from build123d import *

# Parameters (mm, degrees)
SKETCH1_W           = 70.8
SKETCH1_H           = 40
BOSS_EXTRUDE1_DEPTH = 10
SKETCH2_R           = 1.32
CUT_EXTRUDE1_DEPTH  = 11
SKETCH3_R           = 3.4
CUT_EXTRUDE2_DEPTH  = 11
SKETCH4_R           = 5.375
CUT_EXTRUDE3_DEPTH  = 7


with BuildPart() as part:
    # Sketch1 → Boss-Extrude1 (new body)
    with BuildSketch(Plane.XY):
        Rectangle(SKETCH1_W, SKETCH1_H)
    extrude(amount=BOSS_EXTRUDE1_DEPTH)

    # Sketch2 → Cut-Extrude1 (cut, through all)
    with BuildSketch(Plane.XY.offset(10)):
        with Locations((15.875, -15.875)):
            Circle(SKETCH2_R)
        with Locations((-15.875, -15.875)):
            Circle(SKETCH2_R)
        with Locations((-15.875, 15.875)):
            Circle(SKETCH2_R)
        with Locations((15.875, 15.875)):
            Circle(SKETCH2_R)
    extrude(amount=-CUT_EXTRUDE1_DEPTH, mode=Mode.SUBTRACT)

    # Sketch3 → Cut-Extrude2 (cut, through all)
    with BuildSketch(Plane(origin=(0, 0, 0), x_dir=(-1, 0, 0), z_dir=(0, 0, -1))):
        with Locations((-25.4, -12.7)):
            Circle(SKETCH3_R)
        with Locations((0, -12.7)):
            Circle(SKETCH3_R)
        with Locations((25.4, -12.7)):
            Circle(SKETCH3_R)
        with Locations((0, 12.7)):
            Circle(SKETCH3_R)
        with Locations((25.4, 12.7)):
            Circle(SKETCH3_R)
        with Locations((-25.4, 12.7)):
            Circle(SKETCH3_R)
    extrude(amount=-CUT_EXTRUDE2_DEPTH, mode=Mode.SUBTRACT)

    # Sketch4 → Cut-Extrude3 (cut)
    with BuildSketch(Plane(origin=(0, 0, 0), x_dir=(-1, 0, 0), z_dir=(0, 0, -1))):
        with Locations((25.4, -12.7)):
            Circle(SKETCH4_R)
        with Locations((0, -12.7)):
            Circle(SKETCH4_R)
        with Locations((-25.4, -12.7)):
            Circle(SKETCH4_R)
        with Locations((0, 12.7)):
            Circle(SKETCH4_R)
        with Locations((-25.4, 12.7)):
            Circle(SKETCH4_R)
        with Locations((25.4, 12.7)):
            Circle(SKETCH4_R)
    extrude(amount=-CUT_EXTRUDE3_DEPTH, mode=Mode.SUBTRACT)


solid = part.part
Build history of the part. All positions in model axes, mm. A direction names the side the tool comes from. Round coordinates to 2 decimals unless told otherwise and drop trailing zeros. Loops run counter-clockwise (first coordinate to the right, second up) from the corner with the lowest first, then second, coordinate; pieces in that order, holes last. Notation, with made-up numbers: (33.5, 68) -> (45.5, 68) arc R6 cw to (45.5, 75) -> close; hole circle Ø10 at (80.5, -11.75). An arc over 180 degrees is marked (long way). Answer in a Markdown table with one row per item.
Item 1: Which spindle directions (+Z, -Z, +X, -X, +Y, -Y) get a long thin tool onto all of the face, cutting with end or side? Do faces 1 (the cylindrical face through (-30.53, 14.31, 3.45)), 2 (the flat face through (0, 0, 10)). Say none if no direction does.
Answers below:
| item | result |
|---|---|
| face 1 | -Z |
| face 2 | +Z, +X, -X, +Y, -Y |
Item 2: Saw through at C-C (z = 5). State how many separate pieces and enclosed holes the cut face has, and give its area (3 significant figures).
Answers below:
| item | result |
|---|---|
| separate pieces | 1 |
| enclosed holes | 10 |
| area | 2,270 mm² |
Item 3: Pin check, flat tip, straight feed: pin 1 (8.5 mm diameter, centred on x = -0.5, y = -12.5, fed in from -Z). Stop position of the tip, or through.
Answers below:
| item | result |
|---|---|
| pin 1 | stops at z = 7 |
Item 4: Drill centre lines: L1, parallel to Y at x = 25.4, z = 9.4; L2, parallel to Y at x = 1.5, z = 5; L3, parallel to Z at x = -30, y = -14.5. Where is each one in solid material? Low to high. Write a range as [from, to].
Answers below:
| item | result |
|---|---|
| L1 | y = [-20, -16.1], [-9.3, 9.3], [16.1, 20] |
| L2 | y = [-20, -17.86], [-7.54, 7.54], [17.86, 20] |
| L3 | z = [7, 10] |
Item 5: Saw through at B-B (y = 12.7). Write the cut outline in (x, z) (3 decimals), and give its area (3 significant figures).
Answers below:
| item | result |
|---|---|
| outline | (-35.4, 0) -> (-30.775, 0) -> (-30.775, 7) -> (-28.8, 7) -> (-28.8, 10) -> (-35.4, 10) -> close; (-22, 7) -> (-20.025, 7) -> (-20.025, 0) -> (-5.375, 0) -> (-5.375, 7) -> (-3.4, 7) -> (-3.4, 10) -> (-22, 10) -> close; (3.4, 7) -> (5.375, 7) -> (5.375, 0) -> (20.025, 0) -> (20.025, 7) -> (22, 7) -> (22, 10) -> (3.4, 10) -> close; (28.8, 7) -> (30.775, 7) -> (30.775, 0) -> (35.4, 0) -> (35.4, 10) -> (28.8, 10) -> close |
| area | 421 mm² |
Item 6: Saw through at A-A (x = -25.4). Write the cut outline in (y, z) (3 decimals), and give its area (3 significant figures).
Answers below:
| item | result |
|---|---|
| outline | (-20, 0) -> (-18.075, 0) -> (-18.075, 7) -> (-16.1, 7) -> (-16.1, 10) -> (-20, 10) -> close; (-9.3, 7) -> (-7.325, 7) -> (-7.325, 0) -> (7.325, 0) -> (7.325, 7) -> (9.3, 7) -> (9.3, 10) -> (-9.3, 10) -> close; (16.1, 7) -> (18.075, 7) -> (18.075, 0) -> (20, 0) -> (20, 10) -> (16.1, 10) -> close |
| area | 209 mm² |
Item 7: Mould opens along X. For faces 3 (the flat face through (-29, 13, 7)), 4 (the flat face through (0, -20, 5)), 5 (the flat face through (-35.4, 0, 5)), 6 (the flat face through (35.4, 0, 5)) say: +X half, -X half, draft (parallel to the pull), parting line (faces both ways), or undercut.
Answers below:
| item | result |
|---|---|
| face 3 | undercut |
| face 4 | draft |
| face 5 | -X half |
| face 6 | +X half |
Item 8: Saw through at D-D (x = 24). Write the cut outline in (y, z), and give its area (3 significant figures).
Answers below:
| item | result |
|---|---|
| outline | (-20, 0) -> (-17.89, 0) -> (-17.89, 7) -> (-15.8, 7) -> (-15.8, 10) -> (-20, 10) -> close; (-9.6, 7) -> (-7.51, 7) -> (-7.51, 0) -> (7.51, 0) -> (7.51, 7) -> (9.6, 7) -> (9.6, 10) -> (-9.6, 10) -> close; (15.8, 7) -> (17.89, 7) -> (17.89, 0) -> (20, 0) -> (20, 10) -> (15.8, 10) -> close |
| area | 218 mm² |
